Here's how the part is built. I have some questions about the finished solid (model axes, mm). Coordinates: 2 decimals unless noted, no trailing zeros. Order: outer loops, then holes, each group sorted by start corner. A loop starts at its lowest first (then second) coordinate and runs counter-clockwise, first axis right, second up. Notation, with made-up numbers: (-28, 27) - (-12, 27) arc R16 cw to (-12, 45) - close; hole circle Ø5 at (10.5, 42). An arc over 180 degrees is marked (long way). Answer as CSV lines item,"result". Start each with the question number.
Item 1: Imagine slicing it at D-D on y = 0.7. List the corners of the cut face in (x, z) for me.
Item 2: Imagine slicing it at C-C on z = 130. List the corners of the cut face in (x, y) for me, and give its area (3 significant figures).
Item 3: Imagine slicing it at A-A on z = 14. List the corners of the cut face in (x, y) for me.
Item 4: I need wall thicknesses on line 1 (Z direction, x = -14, y = 0.45); line 2 (X direction, y = 0.25, z = 38.5); line 3 (Z direction, x = -1.5, y = 0.4). Which ranges of each line are inside material? Lowest first, please.
Item 5: Imagine slicing it at B-B on x = 0. List the corners of the cut face in (y, z) for me, and give its area (3 significant figures).
Item 6: I'm going to push flat-ended pins straight in: pin 1 (1 mm diameter, centred on y = 0, z = 110, fed in from +X); pin 2 (0.6 mm diameter, centred on y = -1.5, z = 41.5, fed in from +X); pin 3 (0.6 mm diameter, centred on x = 12.5, y = -1.5, fed in from +Z); pin 4 (1.6 mm diameter, centred on x = -0.5, y = 1.5, fed in from +Z). Where does each tip first touch, or does it pass through?
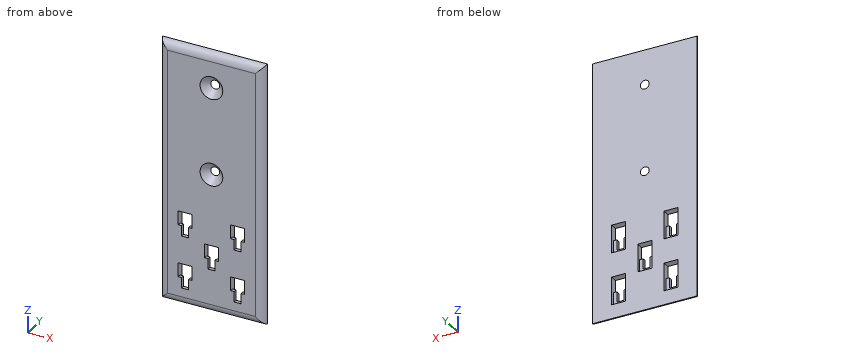
from build123d import *
from build123d import SkipClean  # not in build123d's __all__

# Parameters (mm, degrees)
F0_R        = 1.5
F1_DEPTH    = 2
F0_W        = 2
F0_H        = 6
F0_H_2      = 2
F0_W_2      = 4
F2_DEPTH    = 2
F4_T1_DEPTH = 84.4948974279
F4_T3_DEPTH = 174.4948974279


# Not quite as in the source:
# - a fillet or chamfer that OpenCascade refuses, or shapes differently, is made with other operations: its cross-section is extruded or revolved along the edge and cut away or added


with BuildPart() as f1:
    # F0 (on Front) → F1 (new body)
    with BuildSketch(Plane.XZ):
        with BuildLine():
            Line((-30, 150), (-30, 80))
            Line((-30, 80), (-1.5, 80))
            ThreePointArc((-1.5, 80), (0, 81.5), (1.5, 80))
            Line((1.5, 80), (30, 80))
            Line((30, 80), (30, 150))
            Line((30, 150), (-30, 150))
        make_face()
        with Locations((0, 130)):
            Circle(F0_R, mode=Mode.SUBTRACT)
        with BuildLine():
            Line((-30, 0), (0, 0))
            Line((0, 0), (30, 0))
            Line((30, 0), (30, 80))
            Line((30, 80), (1.5, 80))
            ThreePointArc((1.5, 80), (0, 78.5), (-1.5, 80))
            Line((-1.5, 80), (-30, 80))
            Line((-30, 80), (-30, 0))
        make_face()
        Polygon((-11, 24), (-11, 16), (-11, 10), (-11, 8), (-13, 8), (-17, 8), (-19, 8), (-19, 10), (-19, 16), (-19, 24), align=None, mode=Mode.SUBTRACT)
        Polygon((-11, 48), (-11, 46), (-11, 40), (-11, 38), (-13, 38), (-17, 38), (-19, 38), (-19, 40), (-19, 46), (-19, 48), (-19, 54), (-11, 54), align=None, mode=Mode.SUBTRACT)
        Polygon((4, 39), (4, 31), (4, 25), (4, 23), (2, 23), (-2, 23), (-4, 23), (-4, 25), (-4, 31), (-4, 39), align=None, mode=Mode.SUBTRACT)
        Polygon((19, 24), (19, 16), (19, 10), (19, 8), (17, 8), (13, 8), (11, 8), (11, 10), (11, 16), (11, 24), align=None, mode=Mode.SUBTRACT)
        Polygon((19, 54), (19, 46), (19, 40), (19, 38), (17, 38), (13, 38), (11, 38), (11, 40), (11, 46), (11, 54), align=None, mode=Mode.SUBTRACT)
    extrude(amount=-F1_DEPTH)

    # F0 (on Front) → F2 (join)
    with BuildSketch(Plane.XZ):
        with BuildLine():
            Line((-30, 0), (0, 0))
            Line((0, 0), (30, 0))
            Line((30, 0), (30, 80))
            Line((30, 80), (1.5, 80))
            ThreePointArc((1.5, 80), (0, 78.5), (-1.5, 80))
            Line((-1.5, 80), (-30, 80))
            Line((-30, 80), (-30, 0))
        make_face()
        Polygon((-11, 24), (-11, 16), (-11, 10), (-11, 8), (-13, 8), (-17, 8), (-19, 8), (-19, 10), (-19, 16), (-19, 24), align=None, mode=Mode.SUBTRACT)
        Polygon((-11, 48), (-11, 46), (-11, 40), (-11, 38), (-13, 38), (-17, 38), (-19, 38), (-19, 40), (-19, 46), (-19, 48), (-19, 54), (-11, 54), align=None, mode=Mode.SUBTRACT)
        Polygon((4, 39), (4, 31), (4, 25), (4, 23), (2, 23), (-2, 23), (-4, 23), (-4, 25), (-4, 31), (-4, 39), align=None, mode=Mode.SUBTRACT)
        Polygon((19, 24), (19, 16), (19, 10), (19, 8), (17, 8), (13, 8), (11, 8), (11, 10), (11, 16), (11, 24), align=None, mode=Mode.SUBTRACT)
        Polygon((19, 54), (19, 46), (19, 40), (19, 38), (17, 38), (13, 38), (11, 38), (11, 40), (11, 46), (11, 54), align=None, mode=Mode.SUBTRACT)
        with BuildLine():
            Line((-30, 150), (-30, 80))
            Line((-30, 80), (-1.5, 80))
            ThreePointArc((-1.5, 80), (0, 81.5), (1.5, 80))
            Line((1.5, 80), (30, 80))
            Line((30, 80), (30, 150))
            Line((30, 150), (-30, 150))
        make_face()
        with Locations((0, 130)):
            Circle(F0_R, mode=Mode.SUBTRACT)
        with Locations((-12, 43)):
            Rectangle(F0_W, F0_H)
        with Locations((-12, 39)):
            Rectangle(F0_W, F0_H_2)
        with Locations((-18, 43)):
            Rectangle(F0_W, F0_H)
        with Locations((-15, 39)):
            Rectangle(F0_W_2, F0_H_2)
        with Locations((-18, 39)):
            Rectangle(F0_W, F0_H_2)
        with Locations((18, 43)):
            Rectangle(F0_W, F0_H)
        with Locations((18, 39)):
            Rectangle(F0_W, F0_H_2)
        with Locations((12, 43)):
            Rectangle(F0_W, F0_H)
        with Locations((15, 39)):
            Rectangle(F0_W_2, F0_H_2)
        with Locations((12, 39)):
            Rectangle(F0_W, F0_H_2)
        with Locations((3, 28)):
            Rectangle(F0_W, F0_H)
        with Locations((3, 24)):
            Rectangle(F0_W, F0_H_2)
        with Locations((-3, 28)):
            Rectangle(F0_W, F0_H)
        with Locations((0, 24)):
            Rectangle(F0_W_2, F0_H_2)
        with Locations((-3, 24)):
            Rectangle(F0_W, F0_H_2)
        with Locations((-12, 13)):
            Rectangle(F0_W, F0_H)
        with Locations((-12, 9)):
            Rectangle(F0_W, F0_H_2)
        with Locations((-18, 13)):
            Rectangle(F0_W, F0_H)
        with Locations((-15, 9)):
            Rectangle(F0_W_2, F0_H_2)
        with Locations((-18, 9)):
            Rectangle(F0_W, F0_H_2)
        with Locations((18, 13)):
            Rectangle(F0_W, F0_H)
        with Locations((18, 9)):
            Rectangle(F0_W, F0_H_2)
        with Locations((12, 13)):
            Rectangle(F0_W, F0_H)
        with Locations((15, 9)):
            Rectangle(F0_W_2, F0_H_2)
        with Locations((12, 9)):
            Rectangle(F0_W, F0_H_2)
    with SkipClean():  # cleaning this boolean's faces spoils the solid; the shape is the same uncleaned
        extrude(amount=F2_DEPTH)

    # F3: chamfer of 5 on 2 edges, made by hand

    # F3_s1 → F3_t2 (revolve, cut)
    with BuildSketch(Plane.XY.offset(130)):
        Polygon((6.5, -2), (1.5, 3), (1.5, -2), align=None)
    revolve(axis=Axis((0, -2, 130), (0, -1, 0)), mode=Mode.SUBTRACT)

    # F3_s3 → F3_t4 (revolve, cut)
    with BuildSketch(Plane.XY.offset(80)):
        Polygon((-6.5, -2), (-1.5, 3), (-1.5, -2), align=None)
    revolve(axis=Axis((0, -2, 80), (0, 1, 0)), mode=Mode.SUBTRACT)

    # F4: fillet of radius 5 on 4 edges, made by hand

    # F4_s2 → F4_t1 (cut)
    with BuildSketch(Plane.YZ.offset(-42.2474487139)):
        with BuildLine():
            ThreePointArc((2, 0), (-0.8729833462, 1.7367018254), (-2, 4.8989794856))
            Line((-2, 4.8989794856), (-2, 0))
            Line((-2, 0), (2, 0))
        make_face()
        with BuildLine():
            ThreePointArc((-2, 145.1010205144), (-0.8729833462, 148.2632981746), (2, 150))
            Line((2, 150), (-2, 150))
            Line((-2, 150), (-2, 145.1010205144))
        make_face()
    extrude(amount=F4_T1_DEPTH, mode=Mode.SUBTRACT)

    # F4_s4 → F4_t3 (cut)
    with BuildSketch(Plane.XY.offset(-12.2474487139)):
        with BuildLine():
            ThreePointArc((-30, 2), (-28.2632981746, -0.8729833462), (-25.1010205144, -2))
            Line((-25.1010205144, -2), (-30, -2))
            Line((-30, -2), (-30, 2))
        make_face()
        with BuildLine():
            ThreePointArc((25.1010205144, -2), (28.2632981746, -0.8729833462), (30, 2))
            Line((30, 2), (30, -2))
            Line((30, -2), (25.1010205144, -2))
        make_face()
    extrude(amount=F4_T3_DEPTH, mode=Mode.SUBTRACT)


solid = f1.part
Responses:
1,outline,"(-29.54, 0.46) - (29.54, 0.46) - (29.54, 149.54) - (-29.54, 149.54) - close; hole (-19, 8) - (-11, 8) - (-11, 24) - (-19, 24) - close; hole (-19, 38) - (-11, 38) - (-11, 54) - (-19, 54) - close; hole (-4, 23) - (4, 23) - (4, 39) - (-4, 39) - close; hole circle Ø7.6 at (0, 80); hole circle Ø7.6 at (0, 130); hole (11, 8) - (19, 8) - (19, 24) - (11, 24) - close; hole (11, 38) - (19, 38) - (19, 54) - (11, 54) - close"
2,outline,"(-30, 2) arc R5 ccw to (-25.1, -2) - (-6.5, -2) - (-2.5, 2) - close; (2.5, 2) - (6.5, -2) - (25.1, -2) arc R5 ccw to (30, 2) - close"
2,area,"194 mm^2"
3,outline,"(-30, 2) arc R5 ccw to (-25.1, -2) - (-17, -2) - (-17, 0) - (-19, 0) - (-19, 2) - close; (-13, -2) - (13, -2) - (13, 0) - (11, 0) - (11, 2) - (-11, 2) - (-11, 0) - (-13, 0) - close; (17, -2) - (25.1, -2) arc R5 ccw to (30, 2) - (19, 2) - (19, 0) - (17, 0) - close"
4,line 1,"z = 0.6 to 8, 24 to 38, 54 to 149.4"
4,line 2,"x = -29.28 to -19, -11 to -4, 4 to 11, 19 to 29.28"
4,line 3,"z = 0.63 to 23, 39 to 76.18, 83.82 to 126.18, 133.82 to 149.37"
5,outline,"(-2, 4.9) arc R5 ccw to (2, 0) - (2, 23) - (0, 23) - (0, 25) - (-2, 25) - close; (-2, 39) - (2, 39) - (2, 77.5) - (-2, 73.5) - close; (-2, 86.5) - (2, 82.5) - (2, 127.5) - (-2, 123.5) - close; (-2, 136.5) - (2, 132.5) - (2, 150) arc R5 ccw to (-2, 145.1) - close"
5,area,"458 mm^2"
6,pin 1,"stops at x = 29.43"
6,pin 2,"stops at x = 27.81"
6,pin 3,"stops at z = 147.81"
6,pin 4,"stops at z = 150"
